The listing builds one solid part. Answer for the finished solid, in the listing's coordinates (mm). A direction names the side the tool comes from. Coordinates: 2 decimals unless noted, no trailing zeros. Write each loop counter-clockwise with the first axis right and the second up, starting at its lowest first coordinate (ties: lowest second). Pieces come first, ordered by that corner, then holes.
from build123d import *

# Parameters (mm, degrees)
SZKIC1_R                    = 30
SZKIC1_R_2                  = 26
DODANIE_WYCI_GNI_CIE1_DEPTH = 70
SZKIC2_R                    = 60
SZKIC2_R_2                  = 26
DODANIE_WYCI_GNI_CIE2_DEPTH = 5
SZKIC3_R                    = 5.25
WYTNIJ_WYCI_GNI_CIE1_DEPTH  = 5


with BuildPart() as part:
    # Szkic1 → Dodanie-wyciągnięcie1 (new body)
    with BuildSketch(Plane(origin=(0, 0, 0), x_dir=(0, 0, -1), z_dir=(1, 0, 0))):
        Circle(SZKIC1_R)
        Circle(SZKIC1_R_2, mode=Mode.SUBTRACT)
    extrude(amount=DODANIE_WYCI_GNI_CIE1_DEPTH)

    # Szkic2 → Dodanie-wyciągnięcie2 (add)
    with BuildSketch(Plane(origin=(70, 0, 0), x_dir=(0, 0, -1), z_dir=(1, 0, 0))):
        Circle(SZKIC2_R)
        Circle(SZKIC2_R_2, mode=Mode.SUBTRACT)
    extrude(amount=DODANIE_WYCI_GNI_CIE2_DEPTH)

    # Szkic3 → Wytnij-wyciągnięcie1 (cut)
    with BuildSketch(Plane(origin=(75, 0, 0), x_dir=(0, 0, -1), z_dir=(1, 0, 0))):
        with Locations((-45, 0)):
            Circle(SZKIC3_R)
        with Locations((45, 0)):
            Circle(SZKIC3_R)
        with Locations((0, -45)):
            Circle(SZKIC3_R)
        with Locations((0, 45)):
            Circle(SZKIC3_R)
    extrude(amount=-WYTNIJ_WYCI_GNI_CIE1_DEPTH, mode=Mode.SUBTRACT)


solid = part.part
Q1. Which of the six approach directions +Z, -Z, +X, -X, +Y, -Y give full straight-line access (tool end or side, diameter ignored) to faces 4 (the face through (72.54, 3.55, 48.87)), 5 (the face through (70, 28, -12))?
Answers below:
face 4: +X, -X
face 5: -X
Q2. Find the intervals of material crossed by probe 1 along Y at (x, z) = (71.35, 0); probe 2 along Y at (x, z) = (41.5, 0); probe 3 along X at (y, z) = (13, 30), in increasing order.
Answers below:
probe 1: y = -60 to -50.25, -39.75 to -26, 26 to 39.75, 50.25 to 60
probe 2: y = -30 to -26, 26 to 30
probe 3: x = 70 to 75
Q3. Determine the mould class of faces 1 (the face through (75, -12, -26)), 2 (the face through (36.975, -15.821, 20.633)), 3 (the face through (72.46, 2.64, 59.94)) for opening direction Z: released by +Z, released by -Z, zero draft, split by the parting line, or undercut.
Answers below:
face 1: zero draft
face 2: undercut
face 3: split by the parting line
Q4. The part is cut by section A-A, the plane y = 0. Write down the section's boundary in (x, z), then the cut area to 3 significant figures.
Answers below:
outline: (0, -30) - (70, -30) - (70, -39.75) - (75, -39.75) - (75, -26) - (0, -26) - close; (0, 26) - (75, 26) - (75, 39.75) - (70, 39.75) - (70, 30) - (0, 30) - close; (70, -60) - (75, -60) - (75, -50.25) - (70, -50.25) - close; (70, 50.25) - (75, 50.25) - (75, 60) - (70, 60) - close
area: 795 mm2
Q5. The part is cut by section D-D, the plane y = 45. Write down the section's boundary in (x, z), then the cut area to 3 significant figures.
Answers below:
outline: (70, -39.69) - (75, -39.69) - (75, -5.25) - (70, -5.25) - close; (70, 5.25) - (75, 5.25) - (75, 39.69) - (70, 39.69) - close
area: 344 mm2
Q6. Given pin 1 (17 mm diameter, centred on y = -45, z = 0, fed in from +X); pin 2 (9.5 mm diameter, centred on y = 0, z = -45, fed in from -X); pin 3 (12 mm diameter, centred on y = 45, z = 0, fed in from -X); pin 4 (10 mm diameter, centred on x = 51.5, z = 13.5, fed in from -Y), each flat-ended and moving along its own axis, determine where each tip first touches the part or whether it passes through.
Answers below:
pin 1: stops at x = 75
pin 2: passes through
pin 3: stops at x = 70
pin 4: stops at y = -28.77
Q7. The part is cut by section C-C, the plane z = 41.5. Write down the section's boundary in (x, y), then the cut area to 3 significant figures.
Answers below:
outline: (70, -43.33) - (75, -43.33) - (75, -3.91) - (70, -3.91) - close; (70, 3.91) - (75, 3.91) - (75, 43.33) - (70, 43.33) - close
area: 394 mm2
